Part model, mm, in its own coordinate system. Coordinates: 2 decimals unless noted, no trailing zeros. Write each loop counter-clockwise with the first axis right and the second up, starting at its lowest first coordinate (ties: lowest second). Pieces come first, ordered by that corner, then holes. Notation, with made-up numbers: (-19, 65) -> (-2, 65) arc R17 cw to (-2, 88) -> close; hole circle Ø4 at (57, 65). An arc over 180 degrees is marked (long way). One line per question, with ' | ' between items. Start each with the question number.
Item 1: Saw through at C-C (x = 15). List the corners of the cut face in (y, z).
Item 2: Saw through at B-B (y = 3.45). List the corners of the cut face in (x, z).
Item 3: Saw through at A-A (z = -17). List the corners of the cut face in (x, y), and give its area (3 significant figures).
Item 4: Pin check, flat tip, straight feed: pin 1 (1 mm diameter, centred on y = 2.5, z = 34, fed in from +X). Stop position of the tip, or through.
Item 5: Saw through at D-D (z = -1). List the corners of the cut face in (x, y), and give its area (3 significant figures).
Item 6: Probe probe 1 along Z at (x, y) = (35, 2.7); probe 2 along Z at (x, y) = (17, 2.8); probe 3 along X at (y, z) = (3.85, -8). List the from-to ranges inside material, lowest first. Write a range as [from, to].
from build123d import *

# Parameters (mm, degrees)
BOSS_EXTRUDE1_DEPTH = 2
CHAMFER1_SIZE       = 8
BOSS_EXTRUDE2_DEPTH = 2
SKETCH4_W           = 99.768826376
SKETCH4_H           = 91.588754032
CUT_EXTRUDE1_DEPTH  = 2
SKETCH5_R           = 2.5
CUT_EXTRUDE2_DEPTH  = 2
SKETCH6_W           = 15
SKETCH6_H           = 51.780584955
BOSS_EXTRUDE3_DEPTH = 2
SKETCH7_R           = 2.5
CUT_EXTRUDE3_DEPTH  = 62.071622078
SKETCH8_R           = 3.630325665
SKETCH8_R_2         = 3.812865601
BOSS_EXTRUDE4_DEPTH = 2


with BuildPart() as part:
    # Sketch1 → Boss-Extrude1 (new body)
    with BuildSketch(Plane(origin=(0, 0, 0), x_dir=(1, 0, 0), z_dir=(0, 1, 0))):
        Polygon((-1.782487159, -28.34466675), (33.85093234, -28.34466675), (33.85093234, 27.435918205), (-31.480603593, 27.435918205), (-31.480603593, 2.026433414), (-44.933505709, 2.026433414), (-44.933505709, -41.124585136), (-1.782487159, -41.124585136), align=None)
    extrude(amount=BOSS_EXTRUDE1_DEPTH)

    # Chamfer1
    chamfer1_edges = [part.edges().sort_by_distance(p)[0] for p in [
        (-44.933505709, 1, 41.124585136),
    ]]
    chamfer(chamfer1_edges, length=CHAMFER1_SIZE)

    # Sketch3 → Boss-Extrude2 (add)
    with BuildSketch(Plane(origin=(0, 2, 0), x_dir=(1, 0, 0), z_dir=(0, 1, 0))):
        Polygon((-29.480603593, 25.435918205), (31.85093234, 25.435918205), (31.85093234, -26.34466675), (-3.782487159, -26.34466675), (-3.782487159, -39.124585136), (-36.105078585, -39.124585136), (-42.933505709, -32.296158012), (-42.933505709, 0.026433414), (-29.480603593, 0.026433414), align=None)
    extrude(amount=BOSS_EXTRUDE2_DEPTH)

    # Sketch4 → Cut-Extrude1 (cut)
    with BuildSketch(Plane.XZ):
        Rectangle(SKETCH4_W, SKETCH4_H)
    extrude(amount=-CUT_EXTRUDE1_DEPTH, mode=Mode.SUBTRACT)

    # Sketch5 → Cut-Extrude2 (cut)
    with BuildSketch(Plane(origin=(0, 4, 0), x_dir=(1, 0, 0), z_dir=(0, 1, 0))):
        with Locations(Location((-18.814835626, 18.545625727, 0), (0, 0, 270))):
            Circle(SKETCH5_R)
        with Locations(Location((21.185164374, 18.545625727, 0), (0, 0, 270))):
            Circle(SKETCH5_R)
        with Locations(Location((21.185164374, -19.454374273, 0), (0, 0, 270))):
            Circle(SKETCH5_R)
        with Locations(Location((-29.854835626, -26.529137879, 0), (0, 0, 270))):
            Circle(SKETCH5_R)
    extrude(amount=-CUT_EXTRUDE2_DEPTH, mode=Mode.SUBTRACT)

    # Sketch6 → Boss-Extrude3 (add)
    with BuildSketch(Plane(origin=(0, 4, 0), x_dir=(1, 0, 0), z_dir=(0, 1, 0))):
        with Locations((39.35093234, -0.454374273)):
            Rectangle(SKETCH6_W, SKETCH6_H)
    extrude(amount=-BOSS_EXTRUDE3_DEPTH)

    # Sketch7 → Cut-Extrude3 (cut, through all)
    with BuildSketch(Plane(origin=(0, 4, 0), x_dir=(1, 0, 0), z_dir=(0, 1, 0))):
        with Locations(Location((36.185164374, 18.545625727, 0), (0, 0, 270))):
            Circle(SKETCH7_R)
        with Locations(Location((36.185164374, -19.454374273, 0), (0, 0, 270))):
            Circle(SKETCH7_R)
    extrude(amount=-CUT_EXTRUDE3_DEPTH, mode=Mode.SUBTRACT)

    # Sketch8 → Boss-Extrude4 (add)
    with BuildSketch(Plane(origin=(0, 4, 0), x_dir=(1, 0, 0), z_dir=(0, 1, 0))):
        with Locations((21.185164374, 18.545625727)):
            Circle(SKETCH8_R)
        with Locations((21.185164374, -19.454374273)):
            Circle(SKETCH8_R_2)
    extrude(amount=-BOSS_EXTRUDE4_DEPTH)


solid = part.part
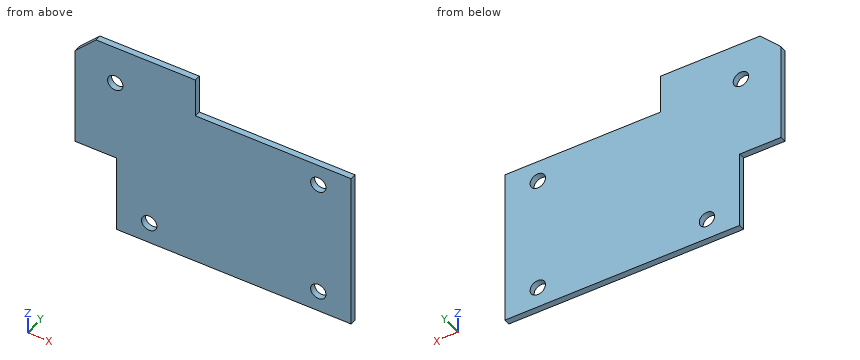
From the geometry:
1) outline: (2, -25.44) -> (4, -25.44) -> (4, 26.34) -> (2, 26.34) -> close
2) outline: (-42.93, -0.03) -> (-29.48, -0.03) -> (-29.48, -25.44) -> (46.85, -25.44) -> (46.85, 26.34) -> (-3.78, 26.34) -> (-3.78, 39.12) -> (-36.11, 39.12) -> (-42.93, 32.3) -> close; hole circle Ø5 at (-29.85, 26.53); hole circle Ø5 at (-18.81, -18.55); hole circle Ø5 at (36.19, -18.55); hole circle Ø5 at (36.19, 19.45)
3) outline: (-29.48, 2) -> (-20.78, 2) -> (-20.78, 4) -> (-29.48, 4) -> close; (-16.85, 2) -> (34.22, 2) -> (34.22, 4) -> (-16.85, 4) -> close; (38.15, 2) -> (46.85, 2) -> (46.85, 4) -> (38.15, 4) -> close | area: 137 mm2
4) pin 1: x = -3.78
5) outline: (-29.48, 2) -> (46.85, 2) -> (46.85, 4) -> (-29.48, 4) -> close | area: 153 mm2
6) probe 1: [-25.44, -20.75], [-16.34, 17.25], [21.66, 26.34] | probe 2: [-25.44, 26.34] | probe 3: [-29.48, 46.85]
